Read the model definition and answer for the solid it produces. Units are mm, in the model's axes. Face numbers are marked on the shaded views. A direction names the side the tool comes from. Give positions to 0.01 mm unless a question says otherwise; leave off trailing zeros. Loops run counter-clockwise (first coordinate to the right, second up) from the corner with the lowest first, then second, coordinate; pieces in that order, holes last. Notation, with made-up numbers: (41.5, -10) - (100.5, -10) arc R19 cw to (100.5, -2) - close; hole circle Ø1 at (-36.5, 25.5). An arc over 180 degrees is marked (long way). Use a Markdown table: item, result. Add a question column.
Item 1: A cutting plane is placed at C-C (x = 80). Determine the outline of the cut face in (y, z), plus the area to 3 significant figures.
Item 2: Consider probe 1 along X at (y, z) = (68.5, 61.5); probe 2 along Z at (x, y) = (58.5, -32). Determine where each line is inside the solid, lowest interval first. Write a range as [from, to].
Item 3: A cutting plane is placed at D-D (z = -18). Determine the outline of the cut face in (x, y), plus the area to 3 significant figures.
Item 4: A cutting plane is placed at A-A (z = 5). Determine the outline of the cut face in (x, y).
Item 5: Which of the six approach directions +Z, -Z, +X, -X, +Y, -Y give full straight-line access (tool end or side, diameter ignored) to the marked faces 1, 2, 3, 4 and 5?
Item 6: Each of these flat-tipped pins is pushed along its axis until it touches: P1, Ø12.5, axis at x = 98.5, y = -2.5, coming from the +Z side; P2, Ø4, axis at x = 76, y = 2.5, coming from the +Z side; P3, Ø12.5, axis at x = 118.5, z = 3, coming from the +Y side. Where does it stop, or does it pass through?
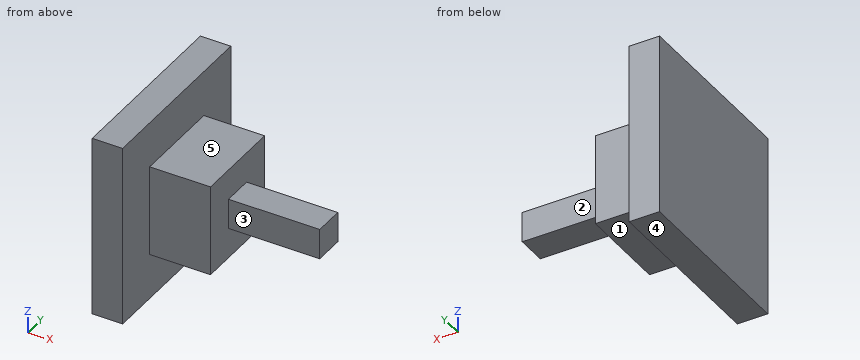
from build123d import *

# Parameters (mm, degrees)
SKETCH1_W           = 25.4
SKETCH1_H           = 25.4
BOSS_EXTRUDE1_DEPTH = 152.4
SKETCH1_3_W         = 76.2
SKETCH1_3_H         = 76.2
SKETCH1_3_W_2       = 25.4
SKETCH1_3_H_2       = 25.4
BOSS_EXTRUDE2_DEPTH = 76.2
SKETCH1_5_W         = 152.4
SKETCH1_5_H         = 152.4
BOSS_EXTRUDE4_DEPTH = 25.4


with BuildPart() as part:
    # Sketch1 → Boss-Extrude1 (new body)
    with BuildSketch(Plane(origin=(0, 0, 0), x_dir=(0, 0, -1), z_dir=(1, 0, 0))):
        Rectangle(SKETCH1_W, SKETCH1_H)
    extrude(amount=BOSS_EXTRUDE1_DEPTH)



with BuildPart() as body_2:
    # Sketch1<3> → Boss-Extrude2 (new body)
    with BuildSketch(Plane(origin=(0, 0, 0), x_dir=(0, 0, -1), z_dir=(1, 0, 0))):
        Rectangle(SKETCH1_3_W, SKETCH1_3_H)
        Rectangle(SKETCH1_3_W_2, SKETCH1_3_H_2, mode=Mode.SUBTRACT)
    extrude(amount=BOSS_EXTRUDE2_DEPTH)


with BuildPart() as part_1:
    add(part.part)

    add(body_2.part)  # Boss-Extrude4 merges body 2
    # Sketch1<5> → Boss-Extrude4 (add)
    with BuildSketch(Plane(origin=(0, 0, 0), x_dir=(0, 0, -1), z_dir=(1, 0, 0))):
        Rectangle(SKETCH1_5_W, SKETCH1_5_H)
    extrude(amount=BOSS_EXTRUDE4_DEPTH)


solid = part_1.part
Geometry says:
| question | item | result |
|---|---|---|
| 1 | outline | (-12.7, -12.7) - (12.7, -12.7) - (12.7, 12.7) - (-12.7, 12.7) - close |
| 1 | area | 645 mm² |
| 2 | probe 1 | [0, 25.4] |
| 2 | probe 2 | [-38.1, 38.1] |
| 3 | outline | (0, -76.2) - (25.4, -76.2) - (25.4, -38.1) - (76.2, -38.1) - (76.2, 38.1) - (25.4, 38.1) - (25.4, 76.2) - (0, 76.2) - close |
| 3 | area | 7,740 mm² |
| 4 | outline | (0, -76.2) - (25.4, -76.2) - (25.4, -38.1) - (76.2, -38.1) - (76.2, -12.7) - (152.4, -12.7) - (152.4, 12.7) - (76.2, 12.7) - (76.2, 38.1) - (25.4, 38.1) - (25.4, 76.2) - (0, 76.2) - close |
| 5 | face 1 | -Z, +X, +Y, -Y |
| 5 | face 2 | +Z, -Z, +X, +Y |
| 5 | face 3 | +Z, -Z, +X, -Y |
| 5 | face 4 | -Z, +X, -X, +Y, -Y |
| 5 | face 5 | +Z, +X, +Y, -Y |
| 6 | P1 | z = 12.7 |
| 6 | P2 | z = 38.1 |
| 6 | P3 | y = 12.7 |
